Input: part model. Units: mm. Frame: model coordinates. Face numbers are marked on the shaded views. A direction names the side the tool comes from. Give positions to 0.01 mm unless a question says otherwise; leave off trailing zeros. Order: outer loops, then holes, each group sorted by start corner. A loop starts at its lowest first (then second) coordinate and runs counter-clockwise, first axis right, second up. Notation, with made-up numbers: (21.5, 22.5) - (59.5, 22.5) arc R17 cw to (59.5, 45.5) - close; hole circle Ø4 at (27, -27.75). An arc over 180 degrees is marked (long way). Answer in a Markdown table with one row per item. Add a question column.
1. Mould query, pull axis Z, two halves, no side actions, for the marked faces 4, 5, 6 and 7. Classes: released by +Z, released by -Z, zero draft, split by the parting line, or undercut.
2. Section query D-D on z = 14. Return loops of the section in (x, y).
3. Section query B-B on y = -2.5. Return loops of the section in (x, z).
4. Section query A-A on z = 10. Return loops of the section in (x, y), and give its area (3 significant figures).
5. Ray query, line 1 (Z direction, x = 0, y = -2.5); line 2 (Y direction, x = -6.75, z = -9.5); line 3 (X direction, y = -5.25, z = 18.5). Return the intervals inside material, ascending. Write a range as [from, to].
6. Section query C-C on x = 0. Return loops of the section in (y, z), and give its area (3 significant figures).
7. Contact query for flat-ended pins moving along their axis: pin 1 (13 mm diameter, centred on x = 0, z = 10, fed in from -Y); pin 2 (1 mm diameter, centred on y = -5, z = 15.5, fed in from -X); pin 3 (5 mm diameter, centred on x = -15, y = -12, fed in from +Z); pin 4 (12 mm diameter, centred on x = 0.5, y = -11, fed in from +Z). Output: stop coordinate, or through.
8. Access query for the marked faces 1, 2 and 3. Directions: +Z, -Z, +X, -X, +Y, -Y. A direction counts if a zero-diameter tool reaches every point of the face in a straight line with its end or side. Return the directions, or none.
```python
from build123d import *

# Parameters (mm, degrees)
F0_R      = 5
F1_DEPTH  = 15
F0_W      = 10
F0_H      = 25
F1_FACE_W = 20
F1_FACE_H = 40
F1_FACE_R = 5
F2_DEPTH  = 20
F3_DEPTH  = 25


with BuildPart() as f1:
    # F0 (on Front) → F1 (new body)
    with BuildSketch(Plane.XZ):
        Polygon((10, -20), (10, 20), (-10, 20), (-10, 5), (-10, -20), align=None)
        with Locations((0, -10)):
            Circle(F0_R, mode=Mode.SUBTRACT)
        with Locations((0, 10)):
            Circle(F0_R, mode=Mode.SUBTRACT)
    extrude(amount=F1_DEPTH)

    # F0 (on Front) + F1_face (on face) → F2 (join)
    with BuildSketch(Plane.XZ):
        Polygon((10, -20), (10, 20), (-10, 20), (-10, 5), (-10, -20), align=None)
        with Locations((0, -10)):
            Circle(F0_R, mode=Mode.SUBTRACT)
        with Locations((0, 10)):
            Circle(F0_R, mode=Mode.SUBTRACT)
        with Locations((-15, -7.5)):
            Rectangle(F0_W, F0_H)
    with BuildSketch(Plane.XZ.offset(15)):
        Rectangle(F1_FACE_W, F1_FACE_H)
        with Locations((0, -10)):
            Circle(F1_FACE_R, mode=Mode.SUBTRACT)
        with Locations((0, 10)):
            Circle(F1_FACE_R, mode=Mode.SUBTRACT)
    extrude(amount=F2_DEPTH)

    # F3 (cut): a face of the model
    f3_faces = [f1.faces().sort_by_distance(p)[0] for p in [
        (0, -35, 0),
    ]]
    extrude(f3_faces, amount=-F3_DEPTH, mode=Mode.SUBTRACT)


solid = f1.part
```
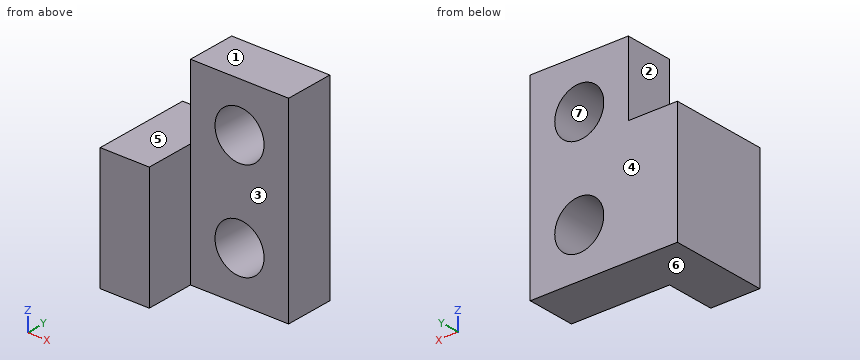
Answer:
| question | item | result |
|---|---|---|
| 1 | face 4 | zero draft |
| 1 | face 5 | released by +Z |
| 1 | face 6 | released by -Z |
| 1 | face 7 | undercut |
| 2 | outline | (-10, -10) - (-3, -10) - (-3, 0) - (-10, 0) - close; (3, -10) - (10, -10) - (10, 0) - (3, 0) - close |
| 3 | outline | (-20, -20) - (10, -20) - (10, 20) - (-10, 20) - (-10, 5) - (-20, 5) - close; hole circle Ø10 at (0, -10); hole circle Ø10 at (0, 10) |
| 4 | outline | (-10, -10) - (-5, -10) - (-5, 0) - (-10, 0) - close; (5, -10) - (10, -10) - (10, 0) - (5, 0) - close |
| 4 | area | 100 mm² |
| 5 | line 1 | z = [-20, -15], [-5, 5], [15, 20] |
| 5 | line 2 | y = [-10, 0] |
| 5 | line 3 | x = [-10, 10] |
| 6 | outline | (-10, -20) - (0, -20) - (0, -15) - (-10, -15) - close; (-10, -5) - (0, -5) - (0, 5) - (-10, 5) - close; (-10, 15) - (0, 15) - (0, 20) - (-10, 20) - close |
| 6 | area | 200 mm² |
| 7 | pin 1 | stops at y = -10 |
| 7 | pin 2 | stops at x = -10 |
| 7 | pin 3 | stops at z = 5 |
| 7 | pin 4 | stops at z = 20 |
| 8 | face 1 | +Z, +X, -X, +Y, -Y |
| 8 | face 2 | +Z, -X, +Y, -Y |
| 8 | face 3 | +Z, -Z, +X, -Y |
